```python
from build123d import *

# Parameters (mm, degrees)
F1_DEPTH = 93
F2_W     = 30.76568
F2_H     = 21.780368
F3_DEPTH = 3


with BuildPart() as f1:
    # F0 (on Top) → F1 (new body)
    with BuildSketch(Plane.XY):
        Polygon((15.92357, 0), (27.581504, 0), (37.5, 17.196862), (37.5, 24), (34.635104, 24), (31.3, 21), (34.5, 21), (34.5, 18), (25.84857, 3), (12.92357, 3), (12.92357, -17), (-12.92407, -17), (-12.92407, 3), (-25.84857, 3), (-34.5, 18), (-34.5, 21), (-31.3, 21), (-34.635104, 24), (-37.5, 24), (-37.5, 17.196862), (-27.581504, 0), (-15.92407, 0), (-15.92407, -20), (-12.92407, -20), (12.92357, -20), (15.92357, -20), align=None)
    extrude(amount=F1_DEPTH)

    # F2 (on Top) → F3 (join)
    with BuildSketch(Plane.XY):
        with Locations((-0.194695, -7.955824)):
            Rectangle(F2_W, F2_H)
    extrude(amount=F3_DEPTH)


solid = f1.part
```
The model under review builds one solid part; all positions refer to its coordinate system, in mm. A direction names the side the tool comes from. Round coordinates to 2 decimals unless told otherwise and drop trailing zeros. Loops run counter-clockwise (first coordinate to the right, second up) from the corner with the lowest first, then second, coordinate; pieces in that order, holes last. Notation, with made-up numbers: (46, -6) - (63, -6) arc R17 ccw to (63, 19) - close; hole circle Ø10 at (23.5, 26). An arc over 180 degrees is marked (long way). Write each question's results on one line, items separated by ' | '. Start each with the question number.
Q1. Take a section at B-B on z = 43. Give the boundary of the cut face in (x, y).
Q2. Take a section at C-C on y = 16. Give the boundary of the cut face in (x, z).
Q3. Tool access review of faces 1 (the flat face through (0, -4, 0)), 2 (the flat face through (34.5, 20, 46)), 3 (the flat face through (0, -17, 47)), 4 (the flat face through (32.99, 22.52, 45.85)): name each direction out of +Z, -Z, +X, -X, +Y, -Y from which nothing blocks a thin tool from reaching the whole face with its end or side.
Q4. Draft analysis for pull direction X (two halves, no side actions). For faces 5 (the flat face through (22, 0, 46)), 6 (the flat face through (15.924, -10, 46)), 7 (the flat face through (19, 3, 46)), 8 (the flat face through (-32.6, 8.7, 45.8)), state which applies: pulls with the +X half, pulls with the -X half, needs draft (parallel to the pull), parting line crosses it, or undercut.
Q5. Take a section at D-D on y = -13. Give the boundary of the cut face in (x, z), plus the area to 3 significant figures.
Q6. Insertion check: P1, Ø1, axis at x = 33, z = 56.5, coming from the -Y side; P2, Ø6, axis at y = -3.5, z = 37.5, coming from the -X side; P3, Ø12, axis at y = -1.5, z = 55, coming from the +X side. Each pin has a flat end and moves straight along its axis. Give the tip position at first contact, or say it passes through.
Q7. Wall thickness on line 1 along X through (y, z) = (-1.5, 61); line 2 along Y through (x, z) = (3, 53); line 3 along Y through (x, z) = (17, 47.5): over which ranges is each line inside the solid? List them lowest first. Write a range as [from, to].
Q8. Take a section at A-A on x = -32.5. Give the boundary of the cut face in (y, z).
Data:
1) outline: (-37.5, 17.2) - (-27.58, 0) - (-15.92, 0) - (-15.92, -20) - (15.92, -20) - (15.92, 0) - (27.58, 0) - (37.5, 17.2) - (37.5, 24) - (34.64, 24) - (31.3, 21) - (34.5, 21) - (34.5, 18) - (25.85, 3) - (12.92, 3) - (12.92, -17) - (-12.92, -17) - (-12.92, 3) - (-25.85, 3) - (-34.5, 18) - (-34.5, 21) - (-31.3, 21) - (-34.64, 24) - (-37.5, 24) - close
2) outline: (-36.81, 0) - (-33.35, 0) - (-33.35, 93) - (-36.81, 93) - close; (33.35, 0) - (36.81, 0) - (36.81, 93) - (33.35, 93) - close
3) face 1: -Z, +X, -X, +Y, -Y | face 2: +Z, -Z | face 3: +Z, +Y | face 4: +Z, -Z, +Y
4) face 5: needs draft | face 6: pulls with the +X half | face 7: undercut | face 8: pulls with the -X half
5) outline: (-15.92, 0) - (15.92, 0) - (15.92, 93) - (12.92, 93) - (12.92, 3) - (-12.92, 3) - (-12.92, 93) - (-15.92, 93) - close | area: 636 mm²
6) P1: stops at y = 8.53 | P2: stops at x = -15.92 | P3: stops at x = 30.18
7) line 1: x = [-15.92, -12.92], [12.92, 15.92] | line 2: y = [-20, -17] | line 3: y = [0, 3]
8) outline: (8.53, 0) - (14.53, 0) - (14.53, 93) - (8.53, 93) - close; (21, 0) - (22.08, 0) - (22.08, 93) - (21, 93) - close
